from build123d import *

# Parameters (mm, degrees)
F0_W     = 14
F0_H     = 22.477162
F1_DEPTH = 5
F2_R     = 6


with BuildPart() as f1:
    # F0 (on Top) → F1 (new body)
    with BuildSketch(Plane.XY):
        Polygon((0, 31.128641), (0, 0), (4.980863, 0), (24, 0), (24, 31.128641), align=None)
        with Locations((11.980863, 16.196262)):
            Rectangle(F0_W, F0_H, mode=Mode.SUBTRACT)
    extrude(amount=F1_DEPTH)

    # F2
    f2_edges = [f1.edges().sort_by_distance(p)[0] for p in [
        (4.980863, 27.434843, 2.5),
        (4.980863, 4.957681, 2.5),
        (18.980863, 4.957681, 2.5),
        (18.980863, 27.434843, 2.5),
    ]]
    fillet(f2_edges, radius=F2_R)


solid = f1.part
Can you work these out from the model? Positions are in its coordinate system, mm. A direction names the side the tool comes from. Give positions to 0.01 mm unless a question says otherwise; leave off trailing zeros. Write each loop counter-clockwise with the first axis right and the second up, starting at its lowest first coordinate (ties: lowest second). Pieces come first, ordered by that corner, then holes. Notation, with made-up numbers: (37.25, 27) -> (46.25, 27) arc R16 cw to (46.25, 50) -> close; hole circle Ø6 at (84.5, 61). An arc over 180 degrees is marked (long way). Answer as a JSON object with one key per item and string values. Group by question number.
Item 1: For faces 4 (the face through (4, 16, 0)), 5 (the face through (17.3, 25.6, 2.5)), which set-ups out of +Z, -Z, +X, -X, +Y, -Y let a thin tool reach every point of the face, with its end or its side?
Item 2: Please list where these lines run through material, in increasing order: line 1 (X direction, y = 14.5, z = 4); line 2 (Y direction, x = 12.5, z = 3.95); line 3 (Y direction, x = 8.25, z = 3.4). Write a range as [from, to].
Item 3: Suppose I cut it at A-A (z = 1.75). Please give me the cut outline in (x, y), plus the area to 3 significant figures.
Item 4: Suppose I cut it at C-C (x = 12.5). Please give me the cut outline in (y, z).
Item 5: We'd pull the mould along Y, two halves only. Please class faces 1 (the face through (12, 27.435, 2)), 2 (the face through (12, 0, 2)), 3 (the face through (0, 16, 2)): +Y half, -Y half, draft (parallel to the pull), parting line (faces both ways), or undercut.
Item 6: Suppose I cut it at B-B (y = 13.5). Please give me the cut outline in (x, z).
Findings:
{
 "1": {"face 4": "-Z, +X, -X, +Y, -Y", "face 5": "+Z, -Z"},
 "2": {"line 1": "x = [0, 4.98], [18.98, 24]", "line 2": "y = [0, 4.96], [27.43, 31.13]", "line 3": "y = [0, 5.62], [26.78, 31.13]"},
 "3": {"outline": "(0, 0) -> (24, 0) -> (24, 31.13) -> (0, 31.13) -> close; hole (4.98, 10.96) arc R6 ccw to (10.98, 4.96) -> (12.98, 4.96) arc R6 ccw to (18.98, 10.96) -> (18.98, 21.43) arc R6 ccw to (12.98, 27.43) -> (10.98, 27.43) arc R6 ccw to (4.98, 21.43) -> close", "area": "463 mm²"},
 "4": {"outline": "(0, 0) -> (4.96, 0) -> (4.96, 5) -> (0, 5) -> close; (27.43, 0) -> (31.13, 0) -> (31.13, 5) -> (27.43, 5) -> close"},
 "5": {"face 1": "undercut", "face 2": "-Y half", "face 3": "draft"},
 "6": {"outline": "(0, 0) -> (4.98, 0) -> (4.98, 5) -> (0, 5) -> close; (18.98, 0) -> (24, 0) -> (24, 5) -> (18.98, 5) -> close"}
}
